Build history of the part. All positions in model axes, mm. Face numbers are marked on the shaded views. A direction names the side the tool comes from. Give positions to 0.01 mm unless a question says otherwise; leave off trailing zeros. Write each loop counter-clockwise with the first axis right and the second up, starting at its lowest first coordinate (ties: lowest second). Pieces come first, ordered by that corner, then holes. Notation, with made-up numbers: (-9, -3.75) - (-5, -3.75) arc R20 cw to (-5, 8.25) - close; hole circle Ø2 at (54.5, 47.5). An arc over 180 degrees is marked (long way). Use one line per item in the form item = value. Start each with the question number.
from build123d import *

# Parameters (mm, degrees)
SKETCH_R                       = 2.25
PAD_DEPTH                      = 12
POCKET_DEPTH                   = 2
SKETCH002_R                    = 2.25
POCKET002_DEPTH                = 20.001
PART_MIRRORING_PLACEMENT_ANGLE = 180


with BuildPart() as pocket002:
    # Sketch → Pad (new body)
    with BuildSketch(Plane.XY):
        Polygon((0, -20), (40, -20), (40, 20), (-20, 20), (-20, 0), (0, 0), align=None)
        with Locations((15, 8)):
            Circle(SKETCH_R, mode=Mode.SUBTRACT)
        with Locations((10, -10)):
            Circle(SKETCH_R, mode=Mode.SUBTRACT)
        with Locations((35, 15)):
            Circle(SKETCH_R, mode=Mode.SUBTRACT)
        with Locations((25, -10)):
            Circle(SKETCH_R, mode=Mode.SUBTRACT)
    extrude(amount=PAD_DEPTH)

    # Sketch001 → Pocket (cut)
    with BuildSketch(Plane.XY.offset(12)):
        with BuildLine():
            Line((46, 10), (26, 10))
            ThreePointArc((26, 10), (22.778175, 17.778175), (15, 21))
            Line((15, 21), (0, 21))
            Line((0, 21), (0, -23))
            Line((0, -23), (46, -23))
            Line((46, -23), (46, -12))
            Line((25.382674, -13.981653), (46, -12))
            ThreePointArc((25.382674, -6.018347), (21, -10), (25.382674, -13.981653))
            Line((25.382674, -6.018347), (46, -8))
            Line((46, -8), (46, 10))
        make_face()
    extrude(amount=-POCKET_DEPTH, mode=Mode.SUBTRACT)

    # Sketch002 → Pocket002 (cut, through all)
    with BuildSketch(Plane.XZ):
        with Locations((-10, 6)):
            Circle(SKETCH002_R)
    extrude(amount=-POCKET002_DEPTH, mode=Mode.SUBTRACT)


with BuildPart() as idler_block_top:
    # Part__Mirroring: instance of Pocket002
    add(pocket002.part.mirror(Plane(origin=(0, 0, 0), x_dir=(0, 1, 0), z_dir=(0, 0, 1))))


with BuildPart() as idler_block_top_1:
    # Part__Mirroring placement: moved
    add(idler_block_top.part.rotate(Axis((0, 0, 0), (1, 0, 0)), PART_MIRRORING_PLACEMENT_ANGLE))


solid = idler_block_top_1.part
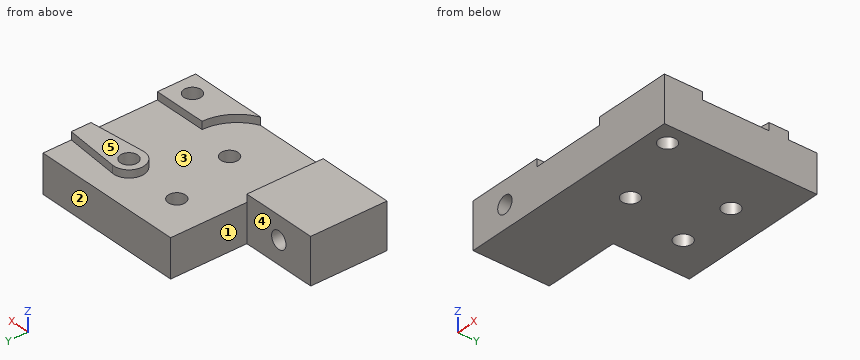
(1) Cut at D-D, the plane x = -10. Give the cut face in (y, z), then the cut area to 3 significant figures.
(2) Pin check, flat tips, straight feed: pin 1 Ø3 at (y, z) = (12, 7) entering from -X; pin 2 Ø2 at (x, z) = (-9.5, 4) entering from +Y; pin 3 Ø2 at (x, z) = (31.5, 11.5) entering from +Y. Stop position of each tip, or through.
(3) Two-plate mould, pull along Y, no slides. Class the marked faces 1, 2 and 3: +Y half, -Y half, draft (parallel to the pull), parting line (faces both ways), or undercut.
(4) Which spindle directions (+Z, -Z, +X, -X, +Y, -Y) get a long thin tool onto all of the face, cutting with end or side? Do the marked faces 4 and 5. Say none if no direction does.
(5) Cut at B-B, the plane x = 10. Give the cut face in (y, z), then the cut area to 3 significant figures.
(6) Cut at C-C, the plane y = -15. Give the cut face in (x, z), then the cut area to 4 significant figures.
(7) Cut at A-A, the plane z = 6. Give the cut face in (x, y).
(8) Wall check: line 1 (X direction, y = 10, z = 6.5); line 2 (Z direction, x = -10, y = -6.75); line 3 (Y direction, x = 15, z = 5). Give the ranges that are in metal, low to high. Write a range as from..to.
Solution:
q1.outline = (-20, 0) - (0, 0) - (0, 3.75) - (-20, 3.75) - close; (-20, 8.25) - (0, 8.25) - (0, 12) - (-20, 12) - close
q1.area = 150 mm2
q2.pin_1 = 0
q2.pin_2 = 0
q2.pin_3 = 13.49
q3.face_1 = draft
q3.face_2 = +Y half
q3.face_3 = undercut
q4.face_4 = +Z, -Z, -X, +Y
q4.face_5 = +Z, +X, -X, +Y, -Y
q5.outline = (-20, 0) - (7.75, 0) - (7.75, 10) - (-20, 10) - close; (12.25, 0) - (20, 0) - (20, 10) - (12.25, 10) - close
q5.area = 355 mm2
q6.outline = (-20, 0) - (32.75, 0) - (32.75, 12) - (24.8, 12) - (24.8, 10) - (0, 10) - (0, 12) - (-20, 12) - close; (37.25, 0) - (40, 0) - (40, 12) - (37.25, 12) - close; hole circle Ø4.5 at (-10, 6)
q6.area = 600.5 mm2
q7.outline = (-20, -20) - (-12.25, -20) - (-12.25, 0) - (-20, 0) - close; (-7.75, -20) - (40, -20) - (40, 20) - (0, 20) - (0, 0) - (-7.75, 0) - close; hole circle Ø4.5 at (10, 10); hole circle Ø4.5 at (15, -8); hole circle Ø4.5 at (25, 10); hole circle Ø4.5 at (35, -15)
q8.line_1 = 0..7.75, 12.25..22.75, 27.25..40
q8.line_2 = 0..3.75, 8.25..12
q8.line_3 = -20..-10.25, -5.75..20
